```python
from build123d import *


with BuildPart() as part:
    # Sketch1 → Carcasa_motor_reductora (revolve)
    with BuildSketch(Plane.XY, mode=Mode.PRIVATE) as carcasa_motor_reductora_sk:
        Polygon((0, 2), (1.8, 2), (1.8, 0), (4.9, 0), (5.5, -0.6), (5.5, -4), (5.15, -4), (5.15, -5), (5.5, -5), (5.5, -30), (4.1, -32), (0, -32), align=None)
    revolve(carcasa_motor_reductora_sk.sketch.rotate(Axis((0, -36, 0), (0, 1, 0)), 90), axis=Axis((0, -36, 0), (0, 1, 0)))


solid = part.part
```
Could you check a few things on this model? Use its own coordinates, in mm. A direction names the side the tool comes from. Round coordinates to 2 decimals unless told otherwise and drop trailing zeros. Loops run counter-clockwise (first coordinate to the right, second up) from the corner with the lowest first, then second, coordinate; pieces in that order, holes last. Notation, with made-up numbers: (10, 51) -> (69, 51) arc R26 cw to (69, 79) -> close; hole circle Ø7 at (58.25, -24.5). An arc over 180 degrees is marked (long way). One line per question, with ' | ' between items.
(1) For pin 1 Ø2 at (x, z) = (-2.5, -1.5) entering from +Y; pin 2 Ø4 at (y, z) = (-24, -4) entering from -X; pin 3 Ø4 at (x, y) = (-3.5, -12) entering from -Z, each with a flat end and sliding along its axis, tell me the tip position at first contact or that it passes through.
Model answer:
pin 1: stops at y = 0 | pin 2: stops at x = -5.12 | pin 3: stops at z = -5.29
(2) For faces 1 (the face through (-0.541, 0.986, -1.717)), 2 (the face through (5.37, -17.68, 1.19)), which set-ups out of +Z, -Z, +X, -X, +Y, -Y let a thin tool reach every point of the face, with its end or its side?
Model answer:
face 1: +Y | face 2: +Y, -Y
(3) If we section it at C-C on y = -25.5: List the corners of the cut face in (x, z) for me.
Model answer:
outline: circle Ø11 at (0, 0)
(4) If we section it at A-A on z = 0: List the corners of the cut face in (x, y) for me.
Model answer:
outline: (-5.5, -30) -> (-4.1, -32) -> (4.1, -32) -> (5.5, -30) -> (5.5, -5) -> (5.15, -5) -> (5.15, -4) -> (5.5, -4) -> (5.5, -0.6) -> (4.9, 0) -> (1.8, 0) -> (1.8, 2) -> (-1.8, 2) -> (-1.8, 0) -> (-4.9, 0) -> (-5.5, -0.6) -> (-5.5, -4) -> (-5.15, -4) -> (-5.15, -5) -> (-5.5, -5) -> close
(5) If I drill on probe 1 along Y at (x, z) = (-1.5, -2.75); probe 2 along X at (y, z) = (-17.5, 2.5); probe 3 along X at (y, z) = (-20, 0.25), over which ranges is the centre line in solid material (lowest first)?
Model answer:
probe 1: y = -32 to 0 | probe 2: x = -4.9 to 4.9 | probe 3: x = -5.49 to 5.49
(6) Thinking about a two-plate mould opening in Y: for faces 3 (the face through (5.37, -2.32, 1.19)), 4 (the face through (3.13, -4.51, 4.09)), 5 (the face through (0, 0, 2)), 6 (the face through (0, -32, 0)), which applies, released by +Y, released by -Y, zero draft, split by the parting line, or undercut?
Model answer:
face 3: zero draft | face 4: undercut | face 5: released by +Y | face 6: released by -Y
(7) If we section it at B-B on x = 0: List the corners of the cut face in (y, z) for me.
Model answer:
outline: (-32, -4.1) -> (-30, -5.5) -> (-5, -5.5) -> (-5, -5.15) -> (-4, -5.15) -> (-4, -5.5) -> (-0.6, -5.5) -> (0, -4.9) -> (0, -1.8) -> (2, -1.8) -> (2, 1.8) -> (0, 1.8) -> (0, 4.9) -> (-0.6, 5.5) -> (-4, 5.5) -> (-4, 5.15) -> (-5, 5.15) -> (-5, 5.5) -> (-30, 5.5) -> (-32, 4.1) -> close
